Verification items for the finished model (mm, model axes). A direction names the side the tool comes from. Coordinates: 2 decimals unless noted, no trailing zeros. Order: outer loops, then holes, each group sorted by start corner. A loop starts at its lowest first (then second) coordinate and runs counter-clockwise, first axis right, second up. Notation, with made-up numbers: (16, 25) -> (25, 25) arc R13 ccw to (25, 36) -> close; hole circle Ø2 at (15, -19). An arc over 180 degrees is marked (long way). Write item = value, one per line. Start each with the question number.
from build123d import *

# Parameters (mm, degrees)
BOSS_EXTRUDE1_DEPTH     = 101
BOSS_EXTRUDE2_DEPTH     = 22
CUT_EXTRUDE1_REACH      = 126.228
CUT_EXTRUDE1_START      = 1
SKETCH3_W               = 3
SKETCH3_H               = 10.606601718
CUT_EXTRUDE2_DEPTH      = 124.228446391
CUT_EXTRUDE2_DEPTH_BACK = 124.228446391


with BuildPart() as part:
    # Sketch1 → Boss-Extrude1 (new body)
    with BuildSketch(Plane(origin=(0, 0, 0), x_dir=(0, 0, -1), z_dir=(1, 0, 0))):
        Polygon((5.303300859, 0), (0, 5.303300859), (-5.303300859, 0), (0, -5.303300859), align=None)
    extrude(amount=BOSS_EXTRUDE1_DEPTH)

    # Sketch2 → Boss-Extrude2 (add)
    with BuildSketch(Plane(origin=(101, 0, 0), x_dir=(0, 0, -1), z_dir=(1, 0, 0))):
        Polygon((0, -5.303300859), (-2.5, -2.803300859), (0, -0.303300859), (2.5, -2.803300859), align=None)
    extrude(amount=BOSS_EXTRUDE2_DEPTH)

    # Sketch3 → Cut-Extrude1 (cut, up to next)
    with BuildSketch(Plane(origin=(0, 0, 0), x_dir=(1, 0, 0), z_dir=(0, 1, 0)).offset(CUT_EXTRUDE1_START), mode=Mode.PRIVATE) as cut_extrude1_sk1:
        with Locations((43, 0)):
            Rectangle(SKETCH3_W, SKETCH3_H)
    cut_extrude1_tool1 = extrude(cut_extrude1_sk1.sketch, amount=CUT_EXTRUDE1_REACH, mode=Mode.PRIVATE) & part.part
    add(cut_extrude1_tool1.solids().sort_by_distance((43, 1, 0))[0], mode=Mode.SUBTRACT)

    # Sketch4 → Cut-Extrude2 (cut, two sides: drawn at the far end of the back side and taken through both)
    with BuildSketch(Plane.XY.offset(-CUT_EXTRUDE2_DEPTH_BACK)):
        Polygon((44.5, 1), (48.803300859, 5.303300859), (44.5, 5.303300859), align=None)
    extrude(amount=CUT_EXTRUDE2_DEPTH + CUT_EXTRUDE2_DEPTH_BACK, mode=Mode.SUBTRACT)


solid = part.part
Item 1: Gauge pin test, flat ends, axial feed: P1, Ø5, axis at x = 73.5, y = 1, coming from the -Z side; P2, Ø2.5, axis at x = 43.5, z = 1, coming from the +Y side; P3, Ø1, axis at x = 44, z = 3.5, coming from the -Y side. Record the tip position at first contact, or that the pin passes through.
Item 2: Section check B-B (y = -1.75). Record the boundary of the cut face in (x, z).
Item 3: Mould release check, pull along X, two halves, no side actions. Record for faces 5 (the flat face through (60.639, -2.689, 2.615)), 6 (the flat face through (0, 0, 0)), 7 (the flat face through (41.5, 3, 0)): pulls with the +X half, pulls with the -X half, needs draft (parallel to the pull), parting line crosses it, or undercut.
Item 4: Section check D-D (x = 8). Record the boundary of the cut face in (y, z), then the cut area to 4 significant figures.
Item 5: Thickness scan on line 1 (X direction, y = -1.25, z = 1.5); line 2 (X direction, y = 4.25, z = 0.75); line 3 (Y direction, x = 31, z = 1). Record the ranges inside material, lowest first.
Item 6: Tool access check on faces 1 (the flat face through (111.846, -1.536, -1.233)), 2 (the flat face through (111.846, -1.571, 1.267)), 3 (the flat face through (43, 1, 0)), 4 (the flat face through (101, 0, 0)). Record the directions out of +Z, -Z, +X, -X, +Y, -Y that give a thin tool (end or side, any length) a straight path to the whole face; none if there is none.
Item 7: Section check C-C (z = 1.5). Record the boundary of the cut face in (x, y), then the cut area to 3 significant figures.
Item 8: Section check A-A (y = 3.25). Record the boundary of the cut face in (x, z), then the cut area to 3 significant figures.
Filled sheet:
q1.P1 = -5.3
q1.P2 = 1.25
q1.P3 = -2.3
q2.outline = (0, -3.55) -> (101, -3.55) -> (101, -1.45) -> (123, -1.45) -> (123, 1.45) -> (101, 1.45) -> (101, 3.55) -> (0, 3.55) -> close
q3.face_5 = needs draft
q3.face_6 = pulls with the -X half
q3.face_7 = undercut
q4.outline = (-5.3, 0) -> (0, -5.3) -> (5.3, 0) -> (0, 5.3) -> close
q4.area = 56.25 mm^2
q5.line_1 = 0 to 101
q5.line_2 = 0 to 41.5, 47.75 to 101
q5.line_3 = -4.3 to 4.3
q6.face_1 = -Z, +X, +Y
q6.face_2 = +Z, +X, +Y
q6.face_3 = +Z, -Z, +Y
q6.face_4 = +X, +Y
q7.outline = (0, -3.8) -> (123, -3.8) -> (123, -1.8) -> (101, -1.8) -> (101, 3.8) -> (47.3, 3.8) -> (44.5, 1) -> (41.5, 1) -> (41.5, 3.8) -> (0, 3.8) -> close
q7.area = 800 mm^2
q8.outline = (0, -2.05) -> (41.5, -2.05) -> (41.5, 2.05) -> (0, 2.05) -> close; (46.75, -2.05) -> (101, -2.05) -> (101, 2.05) -> (46.75, 2.05) -> close
q8.area = 393 mm^2
